from build123d import *

# Parameters (mm, degrees)
SKETCH1_W               = 88.9
SKETCH1_H               = 76.2
BOSS_EXTRUDE1_DEPTH     = 25.4
SKETCH2_R               = 4.1021
CUT_EXTRUDE1_DEPTH      = 19.05
SKETCH5_W               = 88.9
SKETCH5_H               = 0.127
BOSS_EXTRUDE2_DEPTH     = 50.8
SKETCH6_R               = 16.53116582
SKETCH6_R_2             = 8.0645
BOSS_EXTRUDE3_DEPTH     = 50.8
BOSS_EXTRUDE4_DEPTH     = 18.288
SKETCH8_W               = 50.8
SKETCH8_H               = 20.36233164
BOSS_EXTRUDE5_DEPTH     = 27.94
CUT_EXTRUDE6_REACH      = 153.994
CUT_EXTRUDE6_END_RADIUS = 8.0645
SKETCH13_W              = 6.477
SKETCH13_H              = 7.366
CUT_EXTRUDE7_DEPTH      = 22.9616
BOSS_EXTRUDE6_DEPTH     = 50.8
CUT_EXTRUDE8_REACH      = 153.93
SKETCH14_3_R            = 5.25
CUT_EXTRUDE9_DEPTH      = 9
CUT_EXTRUDE10_REACH     = 153.93
SKETCH16_W              = 50.8
SKETCH16_H              = 6.39233418
BOSS_EXTRUDE7_DEPTH     = 50.8
BOSS_EXTRUDE9_START     = 19.05
BOSS_EXTRUDE9_DEPTH     = 19.05
SKETCH22_W              = 7.366
SKETCH22_H              = 12.954
CUT_EXTRUDE15_DEPTH     = 28.4988
MIRROR5_START           = 19.05
MIRROR5_COPY_1_DEPTH    = 19.05
MIRROR5_COPY_2_SKETCH_W = 7.366
MIRROR5_COPY_2_SKETCH_H = 12.954
MIRROR5_COPY_2_DEPTH    = 28.4988
SKETCH25_R              = 5.125
BOSS_EXTRUDE10_DEPTH    = 6.35
SKETCH26_W              = 25.4
SKETCH26_H              = 125.476
CUT_EXTRUDE16_DEPTH     = 6.35
CUT_EXTRUDE17_DEPTH     = 6.35


with BuildPart() as part:
    # Sketch1 → Boss-Extrude1 (new body)
    with BuildSketch(Plane(origin=(0, 0, 0), x_dir=(0, 0, -1), z_dir=(1, 0, 0))):
        with Locations((44.45, 38.1)):
            Rectangle(SKETCH1_W, SKETCH1_H)
    extrude(amount=BOSS_EXTRUDE1_DEPTH)

    # Sketch2 → Cut-Extrude1 (cut)
    with BuildSketch(Plane.ZY):
        with Locations((-85.09, 19.05)):
            Circle(SKETCH2_R)
        with Locations((-3.81, 57.15)):
            Circle(SKETCH2_R)
        with Locations((-3.81, 19.05)):
            Circle(SKETCH2_R)
        with Locations((-85.09, 57.15)):
            Circle(SKETCH2_R)
    extrude(amount=-CUT_EXTRUDE1_DEPTH, mode=Mode.SUBTRACT)

    # Sketch5 → Boss-Extrude2 (add)
    with BuildSketch(Plane(origin=(25.4, 0, 0), x_dir=(0, 0, -1), z_dir=(1, 0, 0))):
        with Locations((44.45, 0.0635)):
            Rectangle(SKETCH5_W, SKETCH5_H)
    extrude(amount=BOSS_EXTRUDE2_DEPTH)

    # Sketch6 → Boss-Extrude3 (add)
    # profile 1 of 2: a face of its own
    with BuildSketch(Plane(origin=(25.4, 0, 0), x_dir=(0, 0, -1), z_dir=(1, 0, 0))):
        with Locations(Location((-1.7145, 38.1635, 0), (0, 0, 275.953033203))):
            Circle(SKETCH6_R)
        with Locations(Location((-1.7145, 38.1635, 0), (0, 0, 77.725329785))):
            Circle(SKETCH6_R_2, mode=Mode.SUBTRACT)
    # profile 2 of 2: a face of its own
    with BuildSketch(Plane(origin=(25.4, 0, 0), x_dir=(0, 0, -1), z_dir=(1, 0, 0))):
        with Locations(Location((90.6145, 38.1635, 0), (0, 0, 264.046966797))):
            Circle(SKETCH6_R)
        with Locations(Location((90.6145, 38.1635, 0), (0, 0, 102.274670215))):
            Circle(SKETCH6_R_2, mode=Mode.SUBTRACT)
    extrude(amount=BOSS_EXTRUDE3_DEPTH)

    # Sketch7 → Boss-Extrude4 (add)
    with BuildSketch(Plane.XY):
        Polygon((76.2, 0.127), (25.4, 0.127), (25.4, 76.2), (0, 76.2), (0, 58.670238274), (19.05, 58.670238274), (19.05, 55.629761726), (0, 55.629761726), (0, 20.570238274), (19.05, 20.570238274), (19.05, 17.529761726), (0, 17.529761726), (0, 0), (76.2, 0), align=None)
    boss_extrude4 = extrude(amount=BOSS_EXTRUDE4_DEPTH)

    # Mirror2: Boss-Extrude4 across plane
    add(boss_extrude4.mirror(Plane.XY.offset(-44.45)))

    # Sketch8 → Boss-Extrude5 (add)
    with BuildSketch(Plane(origin=(0, 0.127, 0), x_dir=(1, 0, 0), z_dir=(0, 1, 0))):
        with Locations((50.8, -1.7145)):
            Rectangle(SKETCH8_W, SKETCH8_H)
    boss_extrude5 = extrude(amount=BOSS_EXTRUDE5_DEPTH)

    # Cut-Extrude6: up to this cylinder (the profile starts outside it)
    cut_extrude6_end = Plane(origin=(57.15, 38.1635, 1.7145), z_dir=(-1, 0, 0)) * Cylinder(CUT_EXTRUDE6_END_RADIUS, 325.117, mode=Mode.PRIVATE)
    # Sketch12 → Cut-Extrude6 (cut, up to the surface)
    with BuildSketch(Plane.XZ, mode=Mode.PRIVATE) as cut_extrude6_sk1:
        with BuildLine():
            ThreePointArc((52.6669, 1.7145), (57.15, -2.7686), (61.6331, 1.7145))
            Line((61.6331, 1.7145), (52.6669, 1.7145))
        make_face()
    cut_extrude6_tool1 = extrude(cut_extrude6_sk1.sketch, amount=-CUT_EXTRUDE6_REACH, mode=Mode.PRIVATE) - cut_extrude6_end
    # Sketch12 → Cut-Extrude6 (cut, up to the surface)
    with BuildSketch(Plane.XZ, mode=Mode.PRIVATE) as cut_extrude6_sk2:
        with BuildLine():
            Line((52.6669, 1.7145), (61.6331, 1.7145))
            ThreePointArc((61.6331, 1.7145), (57.15, 6.1976), (52.6669, 1.7145))
        make_face()
    cut_extrude6_tool2 = extrude(cut_extrude6_sk2.sketch, amount=-CUT_EXTRUDE6_REACH, mode=Mode.PRIVATE) - cut_extrude6_end
    # Sketch12 → Cut-Extrude6 (cut, up to the surface)
    with BuildSketch(Plane.XZ, mode=Mode.PRIVATE) as cut_extrude6_sk3:
        with BuildLine():
            ThreePointArc((52.6669, 1.7145), (57.15, -2.7686), (61.6331, 1.7145))
            Line((61.6331, 1.7145), (52.6669, 1.7145))
        make_face()
    cut_extrude6_tool3 = extrude(cut_extrude6_sk3.sketch, amount=-CUT_EXTRUDE6_REACH, mode=Mode.PRIVATE) - cut_extrude6_end
    # Sketch12 → Cut-Extrude6 (cut, up to the surface)
    with BuildSketch(Plane.XZ, mode=Mode.PRIVATE) as cut_extrude6_sk4:
        with BuildLine():
            Line((52.6669, 1.7145), (61.6331, 1.7145))
            ThreePointArc((61.6331, 1.7145), (57.15, 6.1976), (52.6669, 1.7145))
        make_face()
    cut_extrude6_tool4 = extrude(cut_extrude6_sk4.sketch, amount=-CUT_EXTRUDE6_REACH, mode=Mode.PRIVATE) - cut_extrude6_end
    cut_extrude6 = cut_extrude6_tool1.solids().sort_by_distance((57.15, 0, -0.188187))[0] + cut_extrude6_tool2.solids().sort_by_distance((57.15, 0, 3.617187))[0] + cut_extrude6_tool3.solids().sort_by_distance((57.15, 0, -0.188187))[0] + cut_extrude6_tool4.solids().sort_by_distance((57.15, 0, 3.617187))[0]
    add(cut_extrude6, mode=Mode.SUBTRACT)

    # Sketch13 → Cut-Extrude7 (cut)
    with BuildSketch(Plane.XY.offset(18.288)):
        with Locations((60.3885, 16.383)):
            Rectangle(SKETCH13_W, SKETCH13_H)
        with Locations((53.9115, 16.383)):
            Rectangle(SKETCH13_W, SKETCH13_H)
    cut_extrude7 = extrude(amount=-CUT_EXTRUDE7_DEPTH, mode=Mode.SUBTRACT)

    # Mirror3: Boss-Extrude5, Cut-Extrude6, Cut-Extrude7 across plane
    add(boss_extrude5.mirror(Plane.XY.offset(-44.45)))
    add(cut_extrude6.mirror(Plane.XY.offset(-44.45)), mode=Mode.SUBTRACT)
    add(cut_extrude7.mirror(Plane.XY.offset(-44.45)), mode=Mode.SUBTRACT)

    # Sketch14 → Boss-Extrude6 (add)
    with BuildSketch(Plane(origin=(0, 0.127, 0), x_dir=(1, 0, 0), z_dir=(0, 1, 0))):
        Polygon((48.563230368, 37.763351356), (48.563230368, 51.136648644), (36.981615184, 57.823297288), (25.4, 51.136648644), (25.4, 37.763351356), (36.981615184, 31.076702712), align=None)
        Polygon((28.481615184, 49.357477288), (28.481615184, 39.542522712), (36.981615184, 34.635045424), (45.481615184, 39.542522712), (45.481615184, 49.357477288), (36.981615184, 54.264954576), align=None, mode=Mode.SUBTRACT)
    extrude(amount=BOSS_EXTRUDE6_DEPTH)

    # Sketch14<3> → Cut-Extrude8 (cut, up to next)
    with BuildSketch(Plane(origin=(0, 0.127, 0), x_dir=(1, 0, 0), z_dir=(0, 1, 0)), mode=Mode.PRIVATE) as cut_extrude8_sk1:
        with Locations(Location((36.981615184, 44.45, 0), (0, 0, 270))):
            Circle(SKETCH14_3_R)
    cut_extrude8_tool1 = extrude(cut_extrude8_sk1.sketch, amount=-CUT_EXTRUDE8_REACH, mode=Mode.PRIVATE) & part.part
    add(cut_extrude8_tool1.solids().sort_by_distance((36.981615, 0.127, -44.45))[0], mode=Mode.SUBTRACT)

    # Sketch15 → Cut-Extrude9 (cut)
    with BuildSketch(Plane.XZ):
        Polygon((45.531615184, -39.513655198), (36.981615184, -34.577310397), (28.431615184, -39.513655198), (28.431615184, -49.386344802), (36.981615184, -54.322689603), (45.531615184, -49.386344802), align=None)
    extrude(amount=-CUT_EXTRUDE9_DEPTH, mode=Mode.SUBTRACT)

    # Sketch16 → Cut-Extrude10 (cut, up to next)
    with BuildSketch(Plane(origin=(0, 0.127, 0), x_dir=(1, 0, 0), z_dir=(0, 1, 0)), mode=Mode.PRIVATE) as cut_extrude10_sk1:
        Polygon((48.563230368, 37.763351356), (36.981615184, 31.076702712), (25.4, 31.076702712), (25.4, 8.46666582), (76.2, 8.46666582), (76.2, 80.43333418), (25.4, 80.43333418), (25.4, 57.823297288), (36.981615184, 57.823297288), (48.563230368, 51.136648644), align=None)
    cut_extrude10_tool1 = extrude(cut_extrude10_sk1.sketch, amount=-CUT_EXTRUDE10_REACH, mode=Mode.PRIVATE) & part.part
    # Sketch16 → Cut-Extrude10 (cut, up to next)
    with BuildSketch(Plane(origin=(0, 0.127, 0), x_dir=(1, 0, 0), z_dir=(0, 1, 0)), mode=Mode.PRIVATE) as cut_extrude10_sk2:
        with Locations((50.8, -15.09183291)):
            Rectangle(SKETCH16_W, SKETCH16_H)
    cut_extrude10_tool2 = extrude(cut_extrude10_sk2.sketch, amount=-CUT_EXTRUDE10_REACH, mode=Mode.PRIVATE) & part.part
    # Sketch16 → Cut-Extrude10 (cut, up to next)
    with BuildSketch(Plane(origin=(0, 0.127, 0), x_dir=(1, 0, 0), z_dir=(0, 1, 0)), mode=Mode.PRIVATE) as cut_extrude10_sk3:
        with Locations((50.8, 103.99183291)):
            Rectangle(SKETCH16_W, SKETCH16_H)
    cut_extrude10_tool3 = extrude(cut_extrude10_sk3.sketch, amount=-CUT_EXTRUDE10_REACH, mode=Mode.PRIVATE) & part.part
    add(cut_extrude10_tool1.solids().sort_by_distance((53.397723, 0.127, -44.45))[0], mode=Mode.SUBTRACT)
    add(cut_extrude10_tool2.solids().sort_by_distance((50.8, 0.127, 15.091833))[0], mode=Mode.SUBTRACT)
    add(cut_extrude10_tool3.solids().sort_by_distance((50.8, 0.127, -103.991833))[0], mode=Mode.SUBTRACT)

    # Sketch18 → Boss-Extrude7 (add)
    with BuildSketch(Plane(origin=(0, 0.127, 0), x_dir=(1, 0, 0), z_dir=(0, 1, 0))):
        Polygon((36.981615184, 57.823297288), (25.4, 57.823297288), (25.4, 51.136648644), align=None)
        Polygon((25.4, 37.763351356), (25.4, 31.076702712), (36.981615184, 31.076702712), align=None)
    extrude(amount=BOSS_EXTRUDE7_DEPTH)

    # Sketch20 → Boss-Extrude9 (add)
    with BuildSketch(Plane.ZY.offset(-19.05).offset(BOSS_EXTRUDE9_START)):
        with BuildLine():
            ThreePointArc((0.2921, 19.05), (0.218413175, 18.275976935), (0, 17.529761726))
            Line((0, 17.529761726), (18.288, 17.529761726))
            Line((18.288, 17.529761726), (18.288, 20.570238274))
            Line((18.288, 20.570238274), (0, 20.570238274))
            ThreePointArc((0, 20.570238274), (0.218413175, 19.824023065), (0.2921, 19.05))
        make_face()
    boss_extrude9 = extrude(amount=-BOSS_EXTRUDE9_DEPTH)

    # Sketch22 → Cut-Extrude15 (cut)
    with BuildSketch(Plane.XY.offset(18.288)):
        with Locations((12.1412, 19.05)):
            Rectangle(SKETCH22_W, SKETCH22_H)
    cut_extrude15 = extrude(amount=-CUT_EXTRUDE15_DEPTH, mode=Mode.SUBTRACT)

    # Mirror4: Boss-Extrude9, Cut-Extrude15 across plane
    add(boss_extrude9.mirror(Plane.XY.offset(-44.45)))
    add(cut_extrude15.mirror(Plane.XY.offset(-44.45)), mode=Mode.SUBTRACT)

    # Mirror5: Boss-Extrude9, Cut-Extrude15 across plane
    add(boss_extrude9.mirror(Plane.ZX.offset(38.1)))
    add(cut_extrude15.mirror(Plane.ZX.offset(38.1)), mode=Mode.SUBTRACT)

    # Mirror5 copy 1 sketch → Mirror5 copy 1 (add)
    with BuildSketch(Plane(origin=(19.05, 76.2, -88.9), x_dir=(0, 0, -1), z_dir=(-1, 0, 0)).offset(MIRROR5_START)):
        with BuildLine():
            ThreePointArc((0.2921, 19.05), (0.218413175, 18.275976935), (0, 17.529761726))
            Line((0, 17.529761726), (18.288, 17.529761726))
            Line((18.288, 17.529761726), (18.288, 20.570238274))
            Line((18.288, 20.570238274), (0, 20.570238274))
            ThreePointArc((0, 20.570238274), (0.218413175, 19.824023065), (0.2921, 19.05))
        make_face()
    extrude(amount=-MIRROR5_COPY_1_DEPTH)

    # Mirror5 copy 2 sketch → Mirror5 copy 2 (cut)
    with BuildSketch(Plane(origin=(0, 76.2, -107.188), x_dir=(1, 0, 0), z_dir=(0, 0, -1))):
        with Locations((12.1412, 19.05)):
            Rectangle(MIRROR5_COPY_2_SKETCH_W, MIRROR5_COPY_2_SKETCH_H)
    extrude(amount=-MIRROR5_COPY_2_DEPTH, mode=Mode.SUBTRACT)

    # Sketch25 → Boss-Extrude10 (add)
    with BuildSketch(Plane(origin=(0, 15.350000034, 0), x_dir=(-1, 0, 0), z_dir=(0, -1, 0))):
        Polygon((-36.981615184, 34.577310397), (-28.431615184, 39.513655198), (-28.431615184, 49.386344802), (-36.981615184, 54.322689603), (-45.531615184, 49.386344802), (-45.531615184, 39.513655198), align=None)
        with Locations(Location((-36.981615184, 44.45, 0), (0, 0, 90))):
            Circle(SKETCH25_R, mode=Mode.SUBTRACT)
    extrude(amount=-BOSS_EXTRUDE10_DEPTH)

    # Sketch26 → Cut-Extrude16 (cut)
    with BuildSketch(Plane(origin=(0, 76.2, 0), x_dir=(1, 0, 0), z_dir=(0, 1, 0))):
        with Locations((12.7, 44.45)):
            Rectangle(SKETCH26_W, SKETCH26_H)
    extrude(amount=-CUT_EXTRUDE16_DEPTH, mode=Mode.SUBTRACT)

    # Sketch27 → Cut-Extrude17 (cut)
    with BuildSketch(Plane.XZ):
        Polygon((25.4, -107.188), (25.4, -100.79566582), (76.2, -100.79566582), (76.2, -80.43333418), (25.4, -80.43333418), (25.4, -57.823297288), (36.981615184, -57.823297288), (48.563230368, -51.136648644), (48.563230368, -37.763351356), (36.981615184, -31.076702712), (25.4, -31.076702712), (25.4, -8.46666582), (76.2, -8.46666582), (76.2, 11.89566582), (25.4, 11.89566582), (25.4, 18.288), (0, 18.288), (0, -107.188), align=None)
    extrude(amount=-CUT_EXTRUDE17_DEPTH, mode=Mode.SUBTRACT)


solid = part.part
Input: part model. Units: mm. Frame: model coordinates. A direction names the side the tool comes from. Coordinates: 2 decimals unless noted, no trailing zeros. Loops run counter-clockwise (first coordinate to the right, second up) from the corner with the lowest first, then second, coordinate; pieces in that order, holes last. Notation, with made-up numbers: (78, 70) - (92, 70) arc R29 cw to (92, 103) - close; hole circle Ø11 at (36, 49). An arc over 180 degrees is marked (long way). Answer in a Markdown table with one row per item. Add a question column.
Item 1: Contact query for flat-ended pins moving along their axis: P1, Ø3, axis at y = 51, z = -28, coming from the +X side; P2, Ø8, axis at x = 57.15, z = 1.71, coming from the -Y side; P3, Ø18.5, axis at x = 37.5, z = -49, coming from the +Y side; P4, Ø5, axis at x = 38.5, z = -44.5, coming from the -Y side. Output: stop coordinate, or through.
Item 2: Access query for faces 1 (the flat face through (41.32, 7.66, -37.08)), 2 (the flat face through (8.458, 19, -93)), 3 (the flat face through (25.4, 38, 2)), 4 (the flat face through (8.458, 57, 4)), 5 (the flat face through (28.482, 36, -45)). Directions: +Z, -Z, +X, -X, +Y, -Y. A direction counts if a zero-diameter tool reaches every point of the face in a straight line with its end or side. Return the directions, or none.
Item 3: Section query B-B on z = -44.45. Return the cut outline in (x, y).
Item 4: Line query: line 1 along Z through (x, y) = (4, 19); line 2 along Y through (x, z) = (17, -85). Output: solid intervals per line, ascending. Write a range as [from, to].
Item 5: Mould query, pull axis Z, two halves, no side actions, for faces 6 (the cylindrical face through (52.874, 9.481, -89.268)), 7 (the flat face through (32.77, 7.66, -37.01)), 8 (the flat face through (12, 57, -78.689)), 9 (the flat face through (50.673, 16, -93)). Classes: released by +Z, released by -Z, zero draft, split by the parting line, or undercut.
Item 6: Section query D-D on z = 7.5. Return the cut outline in (x, y).
Item 7: Section query A-A on x = 57.15. State how many separate pieces and enclosed holes the cut face has, then the cut area to 3 significant figures.
Recorded:
| question | item | result |
|---|---|---|
| 1 | P1 | x = 25.4 |
| 1 | P2 | y = 45.16 |
| 1 | P3 | y = 50.93 |
| 1 | P4 | through |
| 2 | face 1 | -Y |
| 2 | face 2 | -Z |
| 2 | face 3 | +X |
| 2 | face 4 | +Z |
| 2 | face 5 | +Y |
| 3 | outline | (0, 6.35) - (28.43, 6.35) - (28.43, 9) - (28.48, 9) - (28.48, 15.35) - (31.86, 15.35) - (31.86, 21.7) - (28.48, 21.7) - (28.48, 50.93) - (25.4, 50.93) - (25.4, 69.85) - (0, 69.85) - close; (42.11, 15.35) - (45.48, 15.35) - (45.48, 9) - (45.53, 9) - (45.53, 6.35) - (48.56, 6.35) - (48.56, 50.93) - (45.48, 50.93) - (45.48, 21.7) - (42.11, 21.7) - close |
| 4 | line 1 | [-107.19, -89.19], [-80.99, -7.91], [0.29, 18.29] |
| 4 | line 2 | [6.35, 14.95], [23.15, 53.05], [61.25, 69.85] |
| 5 | face 6 | undercut |
| 5 | face 7 | undercut |
| 5 | face 8 | released by -Z |
| 5 | face 9 | zero draft |
| 6 | outline | (0, 6.35) - (76.2, 6.35) - (76.2, 32.55) - (25.4, 32.55) - (25.4, 43.78) - (76.2, 43.78) - (76.2, 53.65) - (25.4, 53.65) - (25.4, 69.85) - (0, 69.85) - close; hole (8.46, 12.57) - (15.82, 12.57) - (15.82, 25.53) - (8.46, 25.53) - close; hole (8.46, 50.67) - (15.82, 50.67) - (15.82, 63.63) - (8.46, 63.63) - close; hole (50.67, 12.7) - (63.63, 12.7) - (63.63, 20.07) - (50.67, 20.07) - close |
| 7 | separate pieces | 4 |
| 7 | enclosed holes | 0 |
| 7 | area | 1,430 mm^2 |
